```python
from build123d import *

# Parameters (mm, degrees)
BOSS_EXTRUDE1_DEPTH = 40
CUT_EXTRUDE1_DEPTH  = 40


with BuildPart() as part:
    # Sketch1 → Boss-Extrude1 (new body)
    with BuildSketch(Plane(origin=(0, 0, 0), x_dir=(1, 0, 0), z_dir=(0, 1, 0))):
        Polygon((-18.5, 23.5), (-18.5, -22), (20, -22), (20, -23.5), (-20, -23.5), (-20, 23.5), align=None)
    extrude(amount=BOSS_EXTRUDE1_DEPTH)

    # Sketch2 → Cut-Extrude1 (cut)
    with BuildSketch(Plane.ZY.offset(20)):
        with BuildLine():
            Line((-23.5, 0), (-3.5, 0))
            ThreePointArc((-3.5, 0), (-17.642135624, 5.857864376), (-23.5, 20))
            Line((-23.5, 20), (-23.5, 0))
        make_face()
        with BuildLine():
            Line((-23.5, 40), (-23.5, 20))
            ThreePointArc((-23.5, 20), (-17.642135624, 34.142135624), (-3.5, 40))
            Line((-3.5, 40), (-23.5, 40))
        make_face()
        with BuildLine():
            Line((-10.25, 13.5), (3.75, 13.5))
            ThreePointArc((3.75, 13.5), (10.25, 20), (3.75, 26.5))
            Line((3.75, 26.5), (-10.25, 26.5))
            ThreePointArc((-10.25, 26.5), (-16.75, 20), (-10.25, 13.5))
        make_face()
    extrude(amount=-CUT_EXTRUDE1_DEPTH, mode=Mode.SUBTRACT)


solid = part.part
```
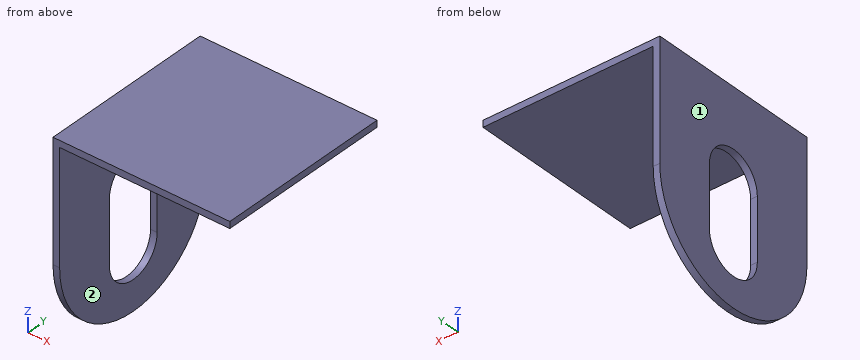
Can you work these out from the model? Positions are in its coordinate system, mm. Face numbers are marked on the shaded views. A direction names the side the tool comes from. Round coordinates to 2 decimals unless told otherwise and drop trailing zeros. Order: outer loops, then holes, each group sorted by start corner. A loop starts at its lowest first (then second) coordinate and runs counter-clockwise, first axis right, second up. Notation, with made-up numbers: (30, -6.75) -> (55, -6.75) arc R25 cw to (55, 8.25) -> close; hole circle Ø11 at (3.5, -26.75). An arc over 180 degrees is marked (long way). Return JSON: item names as keys, results as strings. Group by question number.
1. Which directions (+Z, -Z, +X, -X, +Y, -Y) give clear straight access to the entire face, cutting with the end or side of a thin tool? Please do the marked faces 1 and 2.
2. If we section it at A-A, the plane z = 0.5: Write out the boundary of the cut face in (x, y).
3. If we section it at B-B, the plane y = 21: Write out the boundary of the cut face in (x, z).
4. If we section it at C-C, the plane x = 0: Write out the boundary of the cut face in (y, z).
5. If we section it at D-D, the plane z = -15.5: Write out the boundary of the cut face in (x, y), then the cut area to 3 significant figures.
6. I need wall thicknesses on line 1 (X direction, y = 24.5, z = -15); line 2 (Z direction, x = 5, y = 20.5). Which ranges of each line are inside material? Lowest first, please. Write a range as [from, to].
7. Will these pins go through, and if not, where does the flat tip stop? pin 1 (19 mm diameter, centred on x = -7, y = 22, fed in from -Z); pin 2 (1.2 mm diameter, centred on x = -19, z = -5, fed in from +Y); pin 3 (1 mm diameter, centred on y = 26.5, z = -4, fed in from +X).
Output values:
{
 "1": {"face 1": "+Z, -Z, -X, +Y, -Y", "face 2": "-Z, +X, +Y, -Y"},
 "2": {"outline": "(-20, 0) -> (-18.5, 0) -> (-18.5, 13.5) -> (-20, 13.5) -> close; (-20, 26.5) -> (-18.5, 26.5) -> (-18.5, 40) -> (-20, 40) -> close"},
 "3": {"outline": "(-20, -23.47) -> (-18.5, -23.47) -> (-18.5, -16.67) -> (-20, -16.67) -> close; (-20, 10.17) -> (-18.5, 10.17) -> (-18.5, 22) -> (20, 22) -> (20, 23.5) -> (-20, 23.5) -> close"},
 "4": {"outline": "(0, 22) -> (40, 22) -> (40, 23.5) -> (0, 23.5) -> close"},
 "5": {"outline": "(-20, 4) -> (-18.5, 4) -> (-18.5, 16.17) -> (-20, 16.17) -> close; (-20, 23.83) -> (-18.5, 23.83) -> (-18.5, 36) -> (-20, 36) -> close", "area": "36.5 mm²"},
 "6": {"line 1": "[-20, -18.5]", "line 2": "[22, 23.5]"},
 "7": {"pin 1": "z = 22", "pin 2": "y = 39.98", "pin 3": "x = -18.5"}
}
